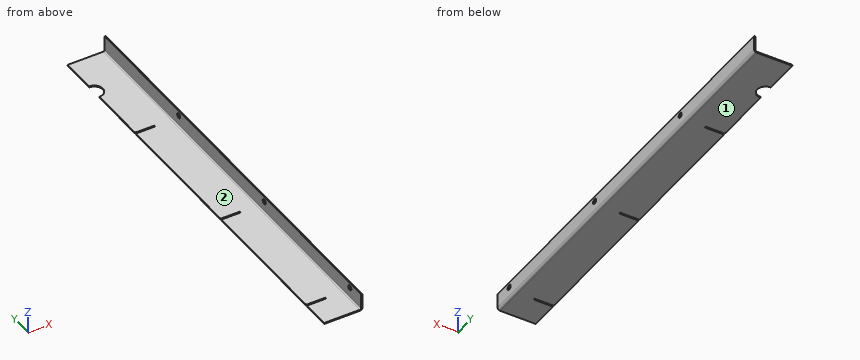
Autodesk Inventor part; units mm, degrees
ref_plane "YZ Plane" through (0, 0, 0) normal (1, 0, 0) x (0, 1, 0)
ref_plane "XZ Plane" through (0, 0, 0) normal (0, 1, 0) x (-1, 0, 0)
ref_plane "XY Plane" through (0, 0, 0) normal (0, 0, 1) x (1, 0, 0)
sketch "Sketch1" plane through (0, 0, 0) normal (0, 0, 1) x (1, 0, 0)
  line L0 (0, 0) -> (-133.9966, 0)
  line L1 (-133.9966, 0) -> (-133.9966, -1489.5)
  line L2 (-133.9966, -1489.5) -> (0, -1489.5)
  line L3 (0, -1489.5) -> (0, 0)
  line L4 (-133.9966, -1389.5) -> (-66, -1389.5)
  line L5 (-66, -1389.5) -> (-66, -1384.5)
  line L6 (-66, -1384.5) -> (-133.9966, -1384.5)
  line L7 (-133.9966, -1384.5) -> (-133.9966, -1389.5)
  line L8 (-133.9966, -893) -> (-66, -893)
  line L9 (-66, -893) -> (-66, -888)
  line L10 (-66, -888) -> (-133.9966, -888)
  line L11 (-133.9966, -888) -> (-133.9966, -893)
  line L12 (-133.9966, -396.5) -> (-66, -396.5)
  line L13 (-66, -396.5) -> (-66, -391.5)
  line L14 (-66, -391.5) -> (-133.9966, -391.5)
  line L15 (-133.9966, -391.5) -> (-133.9966, -396.5)
  circle A0 centre (-133.9966, -154.5) radius 30
  point P0 (-133.9966, -391.5)
  point P1 (-133.9966, -124.5)
  point P2 (-133.9966, -184.5)
  dimension "d0" = 1489.5
  dimension "d1" = 133.9966
  dimension "d2" = 5
  dimension "d4" = 100
  dimension "d7" = 496.5
  dimension "d23" = 66
  dimension "d28" = 60
  dimension "d29" = 1335
extrude "Plate1" add sketch "Sketch1" along normal blind 4 contours L3 L2 L1 L4 L5 L6 L8 L9 L10 L12 L13 L14 A0 L0
sketch "Sketch2" plane through (-4, 0, 0) normal (1, 0, 0) x (0, 1, 0)
  line L0 (-1489.5, 0) -> (0, 0)
  line L1 (0, 0) -> (0, 60)
  line L2 (0, 60) -> (-1489.5, 60)
  line L3 (-1489.5, 60) -> (-1489.5, 0)
edge flange "Flange1" height 60 angle 90 thickness 4 bend radius 4 thickness toward (1, 0, 0) relief tear relief width 4 relief depth 2 edges at (0, -744.75, 4) wall of the first edge with corners at (-4, -1489.5, 0) (-4, 0, 0) (-4, 0, 60) (-4, -1489.5, 60)
bend "Bend1"
corner "Corner1"
chamfer "Corner Chamfer1" distance 3 angle 45 6 edges at (-133.9966, -1389.5, 2) (-133.9966, -1384.5, 2) (-133.9966, -893, 2) (-133.9966, -888, 2) (-133.9966, -391.5, 2) (-133.9966, -396.5, 2)
sketch "Sketch4" plane through (0, -1489.5, 60) normal (1, 0, 0) x (0, 0, -1)
  circle A0 centre (18, 1059.5) radius 9
  line L0 (0, 1489.5) -> (52, 1489.5)
  line L1 (0, 0) -> (0, 1489.5)
  circle A1 centre (18, 562.8333) radius 9
  circle A2 centre (18, 66.1667) radius 9
  point P0 (60, 1489.5)
  dimension "d30" = 430
  dimension "d31" = 18
  dimension "d32" = 18
  dimension "d35" = 496.6667
extrude "Cut1" cut sketch "Sketch4" against normal blind 4
equation "\"d0\" = Стрингер_длина"
equation "\"d1\" = стрингер_глубина_6"
equation "\"d2\" = паз_под_стрингер_толщина"
equation "\"d7\" = 0.333333 * Стрингер_длина"
equation "\"d23\" = паз_под_стрингер_глубина - Thickness"
equation "\"d28\" = 2 * радиус_выреза_под_сварку"
equation "\"d35\" = Шаг_шпангоутов"
equation "\"d40\" = Thickness"
equation "\"d12\" = Thickness"
equation "\"d13\" = BendReliefWidth"
equation "\"d14\" = BendReliefDepth"
equation "\"d15\" = MinimumRemnant"
equation "\"d16\" = TransitionRadius"
equation "\"d17\" = ребро_усилителей"
equation "\"d19\" = BendRadius"
equation "\"d20\" = CornerReliefSize"
equation "\"d21\" = GapSize"
equation "\"d22\" = JacobiRadiusSize"
equation "\"BendRadius\" = Thickness"
equation "\"BendReliefWidth\" = Thickness"
equation "\"BendReliefDepth\" = 0.5 * Thickness"
equation "\"CornerReliefSize\" = 4 * Thickness"
equation "\"MinimumRemnant\" = 2 * Thickness"
equation "\"TransitionRadius\" = BendRadius"
equation "\"JacobiRadiusSize\" = BendRadius"
equation "\"GapSize\" = Thickness"
properties part number "GBK 0204 stringer 6" material "Steel"
Can you work these out from the model? Positions are in its coordinate system, mm. Face numbers are marked on the shaded views. A direction names the side the tool comes from. Coordinates: 2 decimals unless noted, no trailing zeros. Loops run counter-clockwise (first coordinate to the right, second up) from the corner with the lowest first, then second, coordinate; pieces in that order, holes last. Notation, with made-up numbers: (-24, -25.75) - (13, -25.75) arc R27 ccw to (13, 5.25) - close; hole circle Ø11 at (64, -13.75). An arc over 180 degrees is marked (long way). Put each result on its own line as item: value. Start each with the question number.
Item 1: Suppose I cut it at A-A (x = -86.5). Please give me the cut outline in (y, z).
Item 2: For pin 1 (10 mm diameter, centred on x = -72, z = 11, fed in from -Y); pin 2 (4.5 mm diameter, centred on y = -889.5, z = 2, fed in from -X); pin 3 (2 mm diameter, centred on y = -1387, z = 2.5, fed in from -X); pin 4 (23.5 mm diameter, centred on y = -926.67, z = 42, fed in from -X), each with a flat end and sliding along its axis, tell me the tip position at first contact or that it passes through.
Item 3: Suppose I cut it at B-B (z = 42). Please give me the cut outline in (x, y).
Item 4: If I drill on line 1 along Y through (x, z) = (-2.6, 42); line 2 along X through (y, z) = (-904.5, 24); line 3 along Z through (x, y) = (-51.5, -1258), over which ranges is the centre line in solid material (lowest first)?
Item 5: Suppose I cut it at C-C (y = -154.5). Please give me the cut outline in (x, z), and give its area (3 significant figures).
Item 6: Which directions (+Z, -Z, +X, -X, +Y, -Y) give clear straight access to the entire face, cutting with the end or side of a thin tool? Please do the marked faces 1 and 2.
Item 7: Suppose I cut it at D-D (y = -1052.5). Please give me the cut outline in (x, z), and give its area (3 significant figures).
Here are the results:
1. outline: (-1489.5, 0) - (-1389.5, 0) - (-1389.5, 4) - (-1489.5, 4) - close; (-1384.5, 0) - (-893, 0) - (-893, 4) - (-1384.5, 4) - close; (-888, 0) - (-396.5, 0) - (-396.5, 4) - (-888, 4) - close; (-391.5, 0) - (0, 0) - (0, 4) - (-391.5, 4) - close
2. pin 1: through
2. pin 2: x = -131.75
2. pin 3: x = -66
2. pin 4: x = -4
3. outline: (-4, -1489.5) - (0, -1489.5) - (0, -1432.33) - (-4, -1432.33) - close; (-4, -1414.33) - (0, -1414.33) - (0, -935.67) - (-4, -935.67) - close; (-4, -917.67) - (0, -917.67) - (0, -439) - (-4, -439) - close; (-4, -421) - (0, -421) - (0, 0) - (-4, 0) - close
4. line 1: -1489.5 to -1432.33, -1414.33 to -935.67, -917.67 to -439, -421 to 0
4. line 2: -4 to 0
4. line 3: 0 to 4
5. outline: (-104, 0) - (-8, 0) arc R8 ccw to (0, 8) - (0, 60) - (-4, 60) - (-4, 8) arc R4 cw to (-8, 4) - (-104, 4) - close
5. area: 630 mm²
6. face 1: -Z, +X, -X, +Y, -Y
6. face 2: +Z, -X, +Y, -Y
7. outline: (-134, 0) - (-8, 0) arc R8 ccw to (0, 8) - (0, 60) - (-4, 60) - (-4, 8) arc R4 cw to (-8, 4) - (-134, 4) - close
7. area: 750 mm²
